from build123d import *

# Parameters (mm, degrees)
BOSS_EXTRUDE1_DEPTH = 28
SKETCH4_W           = 20
SKETCH4_H           = 28
REVOLVE2_ANGLE      = 180
SKETCH8_W           = 9
SKETCH8_H           = 33.21296959
CUT_EXTRUDE1_DEPTH  = 45
SKETCH9_R           = 5
BOSS_EXTRUDE2_DEPTH = 5


with BuildPart() as part:
    # Sketch1 → Boss-Extrude1 (new body)
    with BuildSketch(Plane.XY):
        with BuildLine():
            Line((0, -225), (40, -225))
            add(Edge.make_bspline(
                [(44.837749122, -20.758189433), (44.837749122, -31.369390936), (28.889425137, -41.782899382), (19.026841833, -81.321540561), (-10.380022908, -166.862499306), (40, -225)],
                knots=[0, 0, 0, 0, 0.243335168, 0.343335168, 1, 1, 1, 1], degree=3))
            ThreePointArc((44.837749122, -20.758189433), (43.585451091, -16.000112379), (40.153070139, -12.475015414))
            Line((40.153070139, -12.475015414), (5.153070139, 8.570056484))
            ThreePointArc((5.153070139, 8.570056484), (-4.922870027, 8.704329423), (-10, 0))
            add(Edge.make_bspline(
                [(-10, 0), (-10, -6.033622411), (-1.935159008, -36.567795894), (2.930618137, -106.909125291), (-14.496902926, -160.944662091), (-10.77837774, -208.408825579), (0, -225)],
                knots=[0, 0, 0, 0, 0.308474866, 0.388557837, 0.800829708, 1, 1, 1, 1], degree=3))
        make_face()
    extrude(amount=BOSS_EXTRUDE1_DEPTH)

    # Sketch4 → Revolve2 (revolve)
    with BuildSketch(Plane.XZ.offset(225)):
        with Locations((30, 14)):
            Rectangle(SKETCH4_W, SKETCH4_H)
    revolve(axis=Axis((20, -225, 28), (0, 0, -1)), revolution_arc=REVOLVE2_ANGLE)

    # Sketch8 → Cut-Extrude1 (cut, symmetric)
    with BuildSketch(Plane(origin=(0, 0, 0), x_dir=(0, 0, -1), z_dir=(1, 0, 0))):
        with Locations((-23.5, -6.606484795)):
            Rectangle(SKETCH8_W, SKETCH8_H)
    cut_extrude1 = extrude(amount=CUT_EXTRUDE1_DEPTH, both=True, mode=Mode.SUBTRACT)

    # Mirror1: Cut-Extrude1 across plane
    add(cut_extrude1.mirror(Plane.XY.offset(14)), mode=Mode.SUBTRACT)

    # Sketch9 → Boss-Extrude2 (add)
    with BuildSketch(Plane.XY.offset(19)):
        with Locations((10.525146493, -7.245327121)):
            Circle(SKETCH9_R)
    boss_extrude2 = extrude(amount=BOSS_EXTRUDE2_DEPTH)

    # Mirror2: Boss-Extrude2 across plane
    add(boss_extrude2.mirror(Plane.XY.offset(14)))


solid = part.part
Geometry check sheet. Reference: the model listing, model coordinates, mm. A direction names the side the tool comes from. Give positions to 0.01 mm unless a question says otherwise; leave off trailing zeros. Answer as a JSON object with one key per item and string values.
(1) Draft check along Y on faces 5 (the cylindrical face through (6.56, -10.29, 6.54)), 6 (the cylindrical face through (43.62, -16.06, 13.93)), 7 (the flat face through (9, -136, 0)), 8 (the cylindrical face through (6.56, -10.29, 21.46)). Enter one of: released by +Y, released by -Y, zero draft, split by the parting line, or undercut.
Report:
{"face 5": "undercut", "face 6": "released by +Y", "face 7": "zero draft", "face 8": "undercut"}
(2) Tool access check on faces 1 (the flat face through (20, -23.213, 4)), 2 (the flat face through (10, -7, 4)), 3 (the flat face through (18, -11, 19)), 4 (the flat face through (20, -23.213, 24)). Record the directions out of +Z, -Z, +X, -X, +Y, -Y that give a thin tool (end or side, any length) a straight path to the whole face; none if there is none.
Report:
{"face 1": "-Z, +X, -X", "face 2": "-Z, +X, -X, +Y", "face 3": "+Z", "face 4": "+Z, +X, -X"}
(3) Depth check by flat-ended pin: pin 1 Ø1.5 at (x, y) = (36.5, -36) entering from -Z; pin 2 Ø5 at (x, z) = (5, 3.5) entering from -Y; pin 3 Ø1.5 at (x, z) = (14.5, 9) entering from +Y; pin 4 Ø12 at (y, z) = (-82.5, 13) entering from +X. Enter the tip coordinate at first touch or a pass-through.
Report:
{"pin 1": "z = 0", "pin 2": "y = -240.61", "pin 3": "y = 3.4", "pin 4": "x = 19.55"}
